from build123d import *

# Parameters (mm, degrees)
BOSS_EXTRUDE1_DEPTH = 11.35
CUT_EXTRUDE1_DEPTH  = 6.35


with BuildPart() as part:
    # Sketch1 → Boss-Extrude1 (new body, symmetric)
    with BuildSketch(Plane.XY):
        Polygon((0, 0), (0, 47), (-17, 47), (-47, 17), (-47, 0), align=None)
    extrude(amount=BOSS_EXTRUDE1_DEPTH, both=True)

    # Sketch2 → Cut-Extrude1 (cut, symmetric)
    with BuildSketch(Plane.XY):
        Polygon((-47, 17), (-47, 2), (-2, 2), (-2, 47), (-17, 47), align=None)
    extrude(amount=CUT_EXTRUDE1_DEPTH, both=True, mode=Mode.SUBTRACT)


solid = part.part
Can you work these out from the model? Positions are in its coordinate system, mm. A direction names the side the tool comes from. Give positions to 0.01 mm unless a question says otherwise; leave off trailing zeros. Order: outer loops, then holes, each group sorted by start corner. A loop starts at its lowest first (then second) coordinate and runs counter-clockwise, first axis right, second up. Notation, with made-up numbers: (1.5, 48) - (10.5, 48) arc R27 cw to (10.5, 80) - close; hole circle Ø8 at (-19, 33). An arc over 180 degrees is marked (long way). Write each question's results on one line, items separated by ' | '.
1) Suppose I cut it at C-C, the plane z = -7.5. Write out the boundary of the cut face in (x, y), then the cut area to 3 significant figures.
Final values:
outline: (-47, 0) - (0, 0) - (0, 47) - (-17, 47) - (-47, 17) - close | area: 1,760 mm^2
2) Suppose I cut it at D-D, the plane z = -4. Write out the boundary of the cut face in (x, y).
Final values:
outline: (-47, 0) - (0, 0) - (0, 47) - (-2, 47) - (-2, 2) - (-47, 2) - close
3) Suppose I cut it at A-A, the plane x = -7.5. Write out the boundary of the cut face in (y, z), then the cut area to 3 significant figures.
Final values:
outline: (0, -11.35) - (47, -11.35) - (47, -6.35) - (2, -6.35) - (2, 6.35) - (47, 6.35) - (47, 11.35) - (0, 11.35) - close | area: 495 mm^2
4) Suppose I cut it at B-B, the plane y = 14.5. Write out the boundary of the cut face in (x, z).
Final values:
outline: (-47, -11.35) - (0, -11.35) - (0, 11.35) - (-47, 11.35) - (-47, 6.35) - (-2, 6.35) - (-2, -6.35) - (-47, -6.35) - close
5) Please list where these lines run through material, in increasing order: line 1 along Z through (x, y) = (-39, 16); line 2 along Y through (x, z) = (-31.5, 1.25); line 3 along X through (y, z) = (13, -4.5). Write a range as [from, to].
Final values:
line 1: z = [-11.35, -6.35], [6.35, 11.35] | line 2: y = [0, 2] | line 3: x = [-2, 0]
6) I'm going to push flat-ended pins straight in: pin 1 Ø8 at (y, z) = (41.5, 7) entering from -X; pin 2 Ø4 at (x, z) = (-21.5, 0.5) entering from +Y. Where does each tip first touch, or does it pass through?
Final values:
pin 1: stops at x = -26.5 | pin 2: stops at y = 2
7) If we mould it in two halves opening along Z, with no side actions, what happens to faces 1 (the face through (-32, 32, 9)), 2 (the face through (-25, 2, 0)), 3 (the face through (-20, 20, 6.35)), 4 (the face through (-19, 19, 11.35))? For each: pulls with the +Z half, pulls with the -Z half, needs draft (parallel to the pull), parting line crosses it, or undercut.
Final values:
face 1: needs draft | face 2: undercut | face 3: undercut | face 4: pulls with the +Z half
8) On a 3-axis mill with a long thin cutter (end or side, diameter ignored), from which of +Z, -Z, +X, -X, +Y, -Y can I reach the whole of each face in a straight line? I mean faces 5 (the face through (-24, 0, 0)), 6 (the face through (-20, 20, -6.35)). Say none if no direction works.
Final values:
face 5: +Z, -Z, +X, -X, -Y | face 6: -X, +Y
